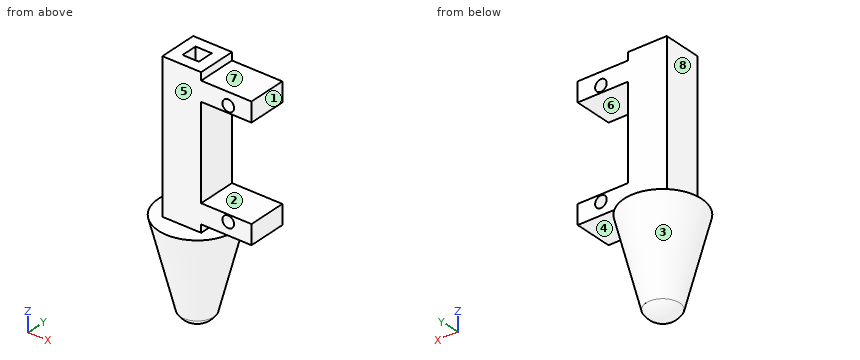
Autodesk Inventor part; units mm, degrees
ref_plane "Work Plane2" through (0, 0, -26) normal (0, 0, 1) x (1, 0, 0)
ref_plane "YZ Plane" through (0, 0, 0) normal (1, 0, 0) x (0, 1, 0)
ref_plane "XZ Plane" through (0, 0, 0) normal (0, 1, 0) x (-1, 0, 0)
sketch "Sketch1" plane through (0, 0, 0) normal (0, 0, 1) x (1, 0, 0)
  line L0 (3.15, -3.15) -> (-3.15, -3.15)
  line L1 (-3.15, -3.15) -> (-3.15, 3.15)
  line L2 (-3.15, 3.15) -> (3.15, 3.15)
  line L3 (3.15, 3.15) -> (3.15, -3.15)
  line L4 (3.15, -3.15) -> (-3.15, 3.15) construction
  line L5 (-3.15, -3.15) -> (3.15, 3.15) construction
  line L6 (5, -5) -> (-5, -5)
  line L7 (-5, -5) -> (-5, 5)
  line L8 (-5, 5) -> (5, 5)
  line L9 (5, 5) -> (5, -5)
  line L10 (5, -5) -> (-5, 5) construction
  line L11 (-5, -5) -> (5, 5) construction
  point P0 (0, 0)
  dimension "d0" = 6.3
  dimension "d1" = 6.3
  dimension "d2" = 10
  dimension "d3" = 10
extrude "Extrusion1" add sketch "Sketch1" along normal mid plane 60
sketch "Sketch3" plane through (0, 0, 0) normal (1, 0, 0) x (0, 1, 0)
  line L0 (5, -30) -> (-5, -30)
  line L1 (0, -30) -> (0, -50)
  line L2 (0, -30) -> (10, -30)
  arc A0 (0, -55) -> (4.3301, -52.5) centre (0, -50) ccw
  line L3 (0, -55) -> (0, -30)
  line L4 (4.3301, -52.5) -> (10, -30)
  point P0 (0, 0)
  dimension "d19" = 20
  dimension "d20" = 10
  dimension "d21" = 10
  dimension "d22" = 5
revolve "Revolution1" add sketch "Sketch3" angle 360 about axis through (0, 0, -30) along (0, 0, -1)
sketch "Sketch4" plane through (0, 0, 0) normal (0, 1, 0) x (-1, 0, 0)
  point P0 (0, 0)
sketch "Sketch5" plane through (0, 0, 0) normal (0, 1, 0) x (-1, 0, 0)
  line L0 (-5, -30) -> (-5, 30)
  line L1 (-5, 0) -> (-5, -23)
  line L2 (-5, 30) -> (-5, -30)
  line L3 (-5, 0) -> (-5, 1)
  line L4 (-5, 1) -> (-5, 6)
  line L5 (-5, 6) -> (-18, 6)
  line L6 (-5, -23) -> (-5, -28)
  line L7 (-5, -28) -> (-18, -28)
  line L8 (-18, -28) -> (-18, -23)
  line L9 (-18, -23) -> (-5, -23)
  line L10 (-5, 1) -> (-18, 1)
  line L11 (-18, 1) -> (-18, 6)
  point P0 (-5, 6)
  point P1 (-5, -28)
  point P2 (-5, -23)
  point P3 (-5, 1)
  dimension "d135" = 23
  dimension "d136" = 1
  dimension "d138" = 13
  dimension "d139" = 5
  dimension "d140" = 13
  dimension "d141" = 5
  dimension "d143" = 5
extrude "Extrusion2" add sketch "Sketch5" along normal mid plane 10
sketch "Sketch7" plane through (-5, -5, 30) normal (0, -1, 0) x (1, 0, 0)
  line L0 (10, 0) -> (10, -60)
  line L1 (23, -53) -> (10, -53)
  line L2 (10, -53) -> (10, -29)
  line L3 (10, -53) -> (10, -29)
  line L4 (10, -29) -> (10, -27.25)
  line L5 (10, -29) -> (23, -29)
  line L6 (10, -27.25) -> (10, -29)
  line L7 (10, -53) -> (10, -54.75)
  line L8 (10, -54.75) -> (17, -54.75)
  line L9 (10, -27.25) -> (17, -27.25)
  circle A0 centre (17, -54.75) radius 1.5
  circle A1 centre (17, -27.25) radius 1.5
  point P0 (10, -23.5)
  point P1 (10, -48.5)
  dimension "d144" = 24
  dimension "d145" = 1.75
  dimension "d146" = 1.75
  dimension "d147" = 7
  dimension "d148" = 7
  dimension "d149" = 3
  dimension "d150" = 3
extrude "Extrusion3" cut sketch "Sketch7" against normal through all
sketch "Sketch19" plane through (0, 0, 30) normal (0, 0, 1) x (1, 0, 0)
  line L0 (0, 0) -> (2.1, 0)
  line L1 (2.1, 0) -> (2.1, -2.1)
  line L2 (2.1, -2.1) -> (-2.1, -2.1)
  line L3 (-2.1, -2.1) -> (-2.1, 2.1)
  line L4 (-2.1, 2.1) -> (2.1, 2.1)
  line L5 (2.1, 2.1) -> (2.1, 0)
  line L6 (3.15, 3.15) -> (-3.15, 3.15)
  line L7 (2.1, 2.1) -> (3.15, 3.15)
  line L8 (3.15, -3.15) -> (3.15, 3.15)
  line L9 (3.15, 3.15) -> (3.15, -3.15)
  line L10 (3.15, -3.15) -> (-3.15, -3.15)
  line L11 (-3.15, -3.15) -> (-3.15, 3.15)
  line L12 (-3.15, 3.15) -> (3.15, 3.15)
  point P0 (-3.15, 3.15)
  dimension "d151" = 2.1
  dimension "d152" = 2.1
  dimension "d153" = 4.2
  dimension "d154" = 4.2
extrude "Extrusion13" add sketch "Sketch19" against normal blind 80
ref_plane "Work Plane2" through (0, 0, -26) normal (0, 0, 1) x (1, 0, 0)
sketch "Sketch22" plane through (-5, -5, 30) normal (0, -1, 0) x (1, 0, 0)
  line L0 (0, -60) -> (0, 0)
  line L1 (10, -24) -> (23, -24)
  line L2 (-4.5508, 0) -> (19.955, 0)
  line L3 (19.955, 0) -> (19.955, -22)
  line L4 (19.955, -22) -> (-10.1203, -22)
  line L5 (-10.1203, -22) -> (-10.1203, 0)
  line L6 (-10.1203, 0) -> (19.955, 0)
  point P0 (5, -30)
  point P1 (0, -31)
  dimension "d176" = 22
extrude "Extrusion16" cut sketch "Sketch22" against normal through all
properties part number "fot"
Here's how the part is built. I have some questions about the finished solid (model axes, mm). Face numbers are marked on the shaded views. A direction names the side the tool comes from. Round coordinates to 2 decimals unless told otherwise and drop trailing zeros. Write each loop counter-clockwise with the first axis right and the second up, starting at its lowest first coordinate (ties: lowest second). Pieces come first, ordered by that corner, then holes.
1. For the marked faces 5, 6, 7 and 8, which set-ups out of +Z, -Z, +X, -X, +Y, -Y let a thin tool reach every point of the face, with its end or its side?
2. I need wall thicknesses on L1, parallel to Z at x = 12, y = 3; L2, parallel to X at y = 1.25, z = -24.75; L3, parallel to Y at x = -1, z = -16.5. Which ranges of each line are inside material? Lowest first, please.
3. Suppose I cut it at B-B (x = 12). List the corners of the cut face in (y, z) for me.
4. Will these pins go through, and if not, where does the flat tip stop? pin 1 Ø2.5 at (x, z) = (12, 2.75) entering from -Y; pin 2 Ø3 at (x, y) = (11, 0) entering from +Z; pin 3 Ø2 at (y, z) = (0.5, -7) entering from +X; pin 4 Ø3.5 at (y, z) = (0.5, -19) entering from -X.
5. Suppose I cut it at A-A (z = 2.75). List the corners of the cut face in (x, y) for me.
6. Suppose I cut it at C-C (z = -21). List the corners of the cut face in (x, y) for me, and give its area (3 significant figures).
7. Suppose I cut it at D-D (y = 3.25). State how many separate pieces and enclosed holes the cut face has, and give its area (3 significant figures).
8. If we mould it in two halves opening along Z, with no side actions, what happens to the marked faces 1, 2, 3 and 4? For each: released by +Z, released by -Z, zero draft, split by the parting line, or undercut.
Answer sheet:
1. face 5: +Z, +X, -X, -Y
1. face 6: +X, +Y, -Y
1. face 7: +Z, +X, +Y, -Y
1. face 8: +Z, -X, +Y, -Y
2. L1: z = -28 to -26.25, -23.25 to -23, 1 to 1.25, 4.25 to 6
2. L2: x = -5 to -2.1, 2.1 to 10.5, 13.5 to 18
2. L3: y = -5 to -2.1, 2.1 to 5
3. outline: (-5, -28) - (5, -28) - (5, -26.25) - (-5, -26.25) - close; (-5, -23.25) - (5, -23.25) - (5, -23) - (-5, -23) - close; (-5, 1) - (5, 1) - (5, 1.25) - (-5, 1.25) - close; (-5, 4.25) - (5, 4.25) - (5, 6) - (-5, 6) - close
4. pin 1: passes through
4. pin 2: stops at z = 6
4. pin 3: stops at x = 5
4. pin 4: stops at x = -5
5. outline: (-5, -5) - (10.5, -5) - (10.5, 5) - (-5, 5) - close; (13.5, -5) - (18, -5) - (18, 5) - (13.5, 5) - close; hole (-2.1, -2.1) - (2.1, -2.1) - (2.1, 2.1) - (-2.1, 2.1) - close
6. outline: (-5, -5) - (5, -5) - (5, 5) - (-5, 5) - close; hole (-2.1, -2.1) - (2.1, -2.1) - (2.1, 2.1) - (-2.1, 2.1) - close
6. area: 82.4 mm2
7. separate pieces: 1
7. enclosed holes: 2
7. area: 785 mm2
8. face 1: zero draft
8. face 2: undercut
8. face 3: released by -Z
8. face 4: undercut
